```python
from build123d import *

# Parameters (mm, degrees)
SKETCH1_R           = 1.45
SKETCH1_R_2         = 5
BOSS_EXTRUDE1_DEPTH = 3
BOSS_EXTRUDE2_DEPTH = 10.5
SKETCH3_R           = 6.75
CUT_EXTRUDE1_DEPTH  = 11.5000001
SKETCH4_R           = 0.9
CUT_EXTRUDE2_DEPTH  = 14.5


with BuildPart() as part:
    # Sketch1 → Boss-Extrude1 (new body)
    with BuildSketch(Plane.XY):
        with BuildLine():
            Line((-14.730127019, -3.5044428), (-4.330127019, 14.508885599))
            ThreePointArc((-4.330127019, 14.508885599), (0, 17.008885599), (4.330127019, 14.508885599))
            Line((4.330127019, 14.508885599), (14.730127019, -3.5044428))
            ThreePointArc((14.730127019, -3.5044428), (14.730127019, -8.5044428), (10.4, -11.0044428))
            Line((10.4, -11.0044428), (-10.4, -11.0044428))
            ThreePointArc((-10.4, -11.0044428), (-14.730127019, -8.5044428), (-14.730127019, -3.5044428))
        make_face()
        with Locations((0, 12.008885599)):
            Circle(SKETCH1_R, mode=Mode.SUBTRACT)
        with Locations((-10.4, -6.0044428)):
            Circle(SKETCH1_R, mode=Mode.SUBTRACT)
        with Locations((10.4, -6.0044428)):
            Circle(SKETCH1_R, mode=Mode.SUBTRACT)
        Circle(SKETCH1_R_2, mode=Mode.SUBTRACT)
    extrude(amount=BOSS_EXTRUDE1_DEPTH)

    # Sketch2 → Boss-Extrude2 (add)
    with BuildSketch(Plane.XY.offset(3)):
        with BuildLine():
            Line((8.030127019, 8.100297611), (11.030127019, 2.904145188))
            add(Edge.make_bspline(
                [(8.030127019, 8.100297611), (-0.869872981, -0.5022214), (11.030127019, 2.904145188)],
                knots=[0, 0, 0, 1, 1, 1], degree=2))
        make_face()
        with BuildLine():
            Line((3, -11.0044428), (-3, -11.0044428))
            add(Edge.make_bspline(
                [(3, -11.0044428), (0, 1.0044428), (-3, -11.0044428)],
                knots=[0, 0, 0, 1, 1, 1], degree=2))
        make_face()
        with BuildLine():
            Line((-11.030127019, 2.904145188), (-8.030127019, 8.100297611))
            add(Edge.make_bspline(
                [(-11.030127019, 2.904145188), (0.869872981, -0.5022214), (-8.030127019, 8.100297611)],
                knots=[0, 0, 0, 1, 1, 1], degree=2))
        make_face()
    extrude(amount=BOSS_EXTRUDE2_DEPTH)

    # Sketch3 → Cut-Extrude1 (cut, through all)
    with BuildSketch(Plane.XY.offset(3)):
        Circle(SKETCH3_R)
    extrude(amount=CUT_EXTRUDE1_DEPTH, mode=Mode.SUBTRACT)

    # Sketch4 → Cut-Extrude2 (cut, through all)
    with BuildSketch(Plane.XY.offset(13.5)):
        with Locations((8.229165125, 4.7511107)):
            Circle(SKETCH4_R)
        with Locations((0, -9.5022214)):
            Circle(SKETCH4_R)
        with Locations((-8.229165125, 4.7511107)):
            Circle(SKETCH4_R)
    extrude(amount=-CUT_EXTRUDE2_DEPTH, mode=Mode.SUBTRACT)


solid = part.part
```
Verification items for the finished model (mm, model axes). A direction names the side the tool comes from. Give positions to 0.01 mm unless a question says otherwise; leave off trailing zeros. Loops run counter-clockwise (first coordinate to the right, second up) from the corner with the lowest first, then second, coordinate; pieces in that order, holes last. Notation, with made-up numbers: M 15,74.25 L 34,74.25 A3 cw 34,78.25 Z; hole C 77.25,17.25 d11. An arc over 180 degrees is marked long. One line per question, with ' | ' between items.
Item 1: Draft check along Y on faces 6 (the face through (-9.13, 4.79, 6.84)), 7 (the face through (-0.12, -8.61, 6.84)), 8 (the face through (0, -11.004, 5)), 9 (the face through (-14.69, -8.57, 1.48)). Enter one of: +Y half, -Y half, draft (parallel to the pull), parting line (faces both ways), or undercut.
Completed:
face 6: undercut | face 7: undercut | face 8: -Y half | face 9: parting line
Item 2: Section check B-B, the plane y = 0. Record the cut outline in (x, z), plus the area to 3 significant figures.
Completed:
outline: M -12.71,0 L -5,0 L -5,3 L -12.71,3 Z; M 5,0 L 12.71,0 L 12.71,3 L 5,3 Z | area: 46.2 mm^2
Item 3: Tool access check on faces 1 (the face through (-1, -9, 13.5)), 2 (the face through (-0.02, -6.75, 8.18)), 3 (the face through (0, -6, 3)), 4 (the face through (5.856, 3.356, 8.177)), 5 (the face through (-0.07, 17.01, 1.48)). Record the directions out of +Z, -Z, +X, -X, +Y, -Y that give a thin tool (end or side, any length) a straight path to the whole face; none if there is none.
Completed:
face 1: +Z, +X, -X, +Y, -Y | face 2: +Z, +Y | face 3: +Z | face 4: +Z, -Y | face 5: +Z, -Z, +Y
Item 4: Section check A-A, the plane x = 0. Record the cut outline in (y, z).
Completed:
outline: M -11,0 L -10.4,0 L -10.4,13.5 L -11,13.5 Z; M -8.6,0 L -5,0 L -5,3 L -6.75,3 L -6.75,13.5 L -8.6,13.5 Z; M 5,0 L 10.56,0 L 10.56,3 L 5,3 Z; M 13.46,0 L 17.01,0 L 17.01,3 L 13.46,3 Z
Item 5: Thickness scan on line 1 (Y direction, x = 9.5, z = 2.5); line 2 (Z direction, x = 4.5, y = -5.5); line 3 (Y direction, x = -0.5, z = 9.5). Record the ranges inside material, lowest first. Write a range as [from, to].
Completed:
line 1: y = [-11, -7.14], [-4.87, 5.55] | line 2: z = [0, 3] | line 3: y = [-11, -10.25], [-8.75, -6.73]
Item 6: Section check C-C, the plane y = -5.5. Record the cut outline in (x, z).
Completed:
outline: M -15.37,0 L -11.76,0 L -11.76,3 L -15.37,3 Z; M -9.04,0 L 9.04,0 L 9.04,3 L -9.04,3 Z; M 11.76,0 L 15.37,0 L 15.37,3 L 11.76,3 Z
Item 7: Depth check by flat-ended pin: P1, Ø11.5, axis at x = 0, y = 0, coming from the +Z side; P2, Ø1, axis at x = 11.5, z = 6.5, coming from the +Y side; P3, Ø1, axis at x = 9, z = 8.5, coming from the +Y side. Enter the tip coordinate at first touch or a pass-through.
Completed:
P1: stops at z = 3 | P2: stops at y = 2.96 | P3: stops at y = 7.29
Item 8: Section check D-D, the plane z = 12.5. State how many separate pieces and enclosed holes the cut face has, plus the area to 3 significant figures.
Completed:
separate pieces: 3 | enclosed holes: 3 | area: 53.7 mm^2
